from build123d import *

# Parameters (mm, degrees)
F0_W        = 73
F0_H        = 40
F1_DEPTH    = 26.5
F0_W_2      = 79
F0_H_2      = 42
F2_DEPTH    = 1.5
F3_W        = 12
F3_H        = 12
F4_DEPTH    = 2
F5_W        = 12
F5_H        = 12
F6_DEPTH    = 2
F7_T        = 2.5
F7_T3_DEPTH = 78
F7_T5_DEPTH = 45
F7_T7_DEPTH = 17
F7_T9_DEPTH = 17


# Not quite as in the source:
# - a shell that OpenCascade refuses in one call is made with other operations: the cavity is built on its own and cut out


with BuildPart() as f1:
    # F0 (on Front) → F1 (new body)
    with BuildSketch(Plane.XZ):
        Rectangle(F0_W, F0_H)
    extrude(amount=F1_DEPTH)

    # F0 (on Front) → F2 (join)
    with BuildSketch(Plane.XZ):
        Rectangle(F0_W_2, F0_H_2)
        Rectangle(F0_W, F0_H, mode=Mode.SUBTRACT)
    extrude(amount=F2_DEPTH)

    # F3 (on face) → F4 (join)
    with BuildSketch(Plane(origin=(-36.5, 0, 0), x_dir=(0, -1, 0), z_dir=(-1, 0, 0))):
        with Locations((7.75, 0)):
            Rectangle(F3_W, F3_H)
    extrude(amount=F4_DEPTH)

    # F5 (on face) → F6 (join)
    with BuildSketch(Plane.YZ.offset(36.5)):
        with Locations((-7.75, 0)):
            Rectangle(F5_W, F5_H)
    extrude(amount=F6_DEPTH)

    # F7: shell of thickness 2.5, made by hand


with BuildPart() as f7_core1:
    # F7_t2: copy of F1
    add(f1.part)

    # the walls: a layer under each face that stays
    f7_faces = [f7_core1.faces().sort_by_distance(p)[0] for p in [
        (0, -14, -20),
        (-36.8666666667, -1.5, -19.6),
        (36.5, -14, 0),
        (-36.5, -14, 0),
        (0, -0.75, -21),
        (39.5, -0.75, 0),
        (0, -0.75, 21),
        (-39.5, -0.75, 0),
        (0, -14, 20),
        (37.5, -13.75, 0),
        (37.5, -7.75, 6),
        (37.5, -1.75, 0),
        (37.5, -7.75, -6),
        (-37.5, -1.75, 0),
        (-37.5, -7.75, 6),
        (-37.5, -13.75, 0),
        (-37.5, -7.75, -6),
        (0, 0, 0),
        (38.5, -7.75, 0),
        (-38.5, -7.75, 0),
    ]]
    thicken(f7_faces, amount=-F7_T, mode=Mode.SUBTRACT)

    # F7_s4 → F7_t3 (cut)
    with BuildSketch(Plane.YZ.offset(-39)):
        Polygon((-1.525, -20.025), (-1.5, -17.5), (1, -17.5), (1, -20), align=None)
        Polygon((-1.525, 20.025), (1, 20), (1, 17.5), (-1.5, 17.5), align=None)
    extrude(amount=F7_T3_DEPTH, mode=Mode.SUBTRACT)

    # F7_s6 → F7_t5 (cut)
    with BuildSketch(Plane.XY.offset(-22.5)):
        Polygon((36.525, -1.525), (36.5, 1), (34, 1), (34, -1.5), align=None)
        Polygon((-36.525, -1.525), (-36.5, 1), (-34, 1), (-34, -1.5), align=None)
    extrude(amount=F7_T5_DEPTH, mode=Mode.SUBTRACT)

    # F7_s8 → F7_t7 (cut)
    with BuildSketch(Plane.XY.offset(-8.5)):
        Polygon((36.525, -13.775), (34, -13.75), (34, -11.25), (36.5, -11.25), align=None)
        Polygon((36.525, -1.725), (34, -1.75), (34, -4.25), (36.5, -4.25), align=None)
        Polygon((-36.525, -1.725), (-34, -1.75), (-34, -4.25), (-36.5, -4.25), align=None)
        Polygon((-36.525, -13.775), (-34, -13.75), (-34, -11.25), (-36.5, -11.25), align=None)
    extrude(amount=F7_T7_DEPTH, mode=Mode.SUBTRACT)

    # F7_s10 → F7_t9 (cut)
    with BuildSketch(Plane.XZ.offset(-0.75)):
        Polygon((36.525, 6.025), (34, 6), (34, 3.5), (36.5, 3.5), align=None)
        Polygon((36.525, -6.025), (34, -6), (34, -3.5), (36.5, -3.5), align=None)
        Polygon((-36.525, 6.025), (-34, 6), (-34, 3.5), (-36.5, 3.5), align=None)
        Polygon((-36.525, -6.025), (-34, -6), (-34, -3.5), (-36.5, -3.5), align=None)
    extrude(amount=F7_T9_DEPTH, mode=Mode.SUBTRACT)


with BuildPart() as f1_1:
    add(f1.part)

    # what is left inside the walls is the cavity
    f7_cavity = [f7_core1.part.solids().sort_by_distance(p)[0] for p in [
        (0, -2.525, -5.833333),
    ]]
    add(f7_cavity, mode=Mode.SUBTRACT)


solid = f1_1.part
Can you work these out from the model? Positions are in its coordinate system, mm. A direction names the side the tool comes from. Round coordinates to 2 decimals unless told otherwise and drop trailing zeros. Loops run counter-clockwise (first coordinate to the right, second up) from the corner with the lowest first, then second, coordinate; pieces in that order, holes last. Notation, with made-up numbers: (-12, -30.75) - (-3, -30.75) arc R25 cw to (-3, 2.25) - close; hole circle Ø4 at (3.5, 47). An arc over 180 degrees is marked (long way). Answer in a Markdown table with one row per item. Add a question column.
Q1. For pin 1 Ø8 at (x, y) = (12, -10.5) entering from +Z; pin 2 Ø1 at (y, z) = (-23, 15) entering from -X; pin 3 Ø2 at (x, z) = (37.5, -1.5) entering from +Y; pin 4 Ø0.6 at (x, y) = (-37, -10) entering from +Z, each with a flat end and sliding along its axis, tell me the tip position at first contact or that it passes through.
Q2. I want a section at A-A on x = -28. List the corners of the cut face in (y, z) for me, and give its area (3 significant figures).
Q3. I need wall thicknesses on L1, parallel to X at y = -12, z = 12; L2, parallel to Z at x = 3, y = -10.25; L3, parallel to X at y = -13, z = 5.5. Which ranges of each line are inside material? Lowest first, please.
Q4. We'd pull the mould along Y, two halves only. Please class faces 1 (the flat face through (0, -2.5, 0)), 2 (the flat face through (-35, -11.25, 0)), 3 (the flat face through (-1, -1, -21)): pulls with the +Y half, pulls with the -Y half, needs draft (parallel to the pull), parting line crosses it, or undercut.
Q5. I want a section at D-D on y = -3.25. List the corners of the cut face in (x, z) for me.
Q6. Which directions (+Z, -Z, +X, -X, +Y, -Y) give clear straight access to the entire face, cutting with the end or side of a thin tool? Please do faces 4 (the flat face through (38.5, -8, 0)), 5 (the flat face through (0, -14, -17.5)), 6 (the flat face through (-37, -8, -6)), 7 (the flat face through (-37, -13.75, 0)), 8 (the flat face through (-35, -8, 3.5)).
Q7. I want a section at C-C on z = 0. List the corners of the cut face in (x, y) for me.
Q8. I want a section at B-B on y = -15. List the corners of the cut face in (x, z) for me, and give its area (3 significant figures).
A:
| question | item | result |
|---|---|---|
| 1 | pin 1 | z = 20 |
| 1 | pin 2 | x = -36.5 |
| 1 | pin 3 | y = 0 |
| 1 | pin 4 | z = 6 |
| 2 | outline | (-26.5, -20) - (-1.5, -20) - (-1.5, -21) - (0, -21) - (0, 21) - (-1.5, 21) - (-1.5, 20) - (-26.5, 20) - (-26.5, 17.5) - (-2.5, 17.5) - (-2.5, -17.5) - (-26.5, -17.5) - close |
| 2 | area | 223 mm^2 |
| 3 | L1 | -36.5 to -34, 34 to 36.5 |
| 3 | L2 | -20 to -17.5, 17.5 to 20 |
| 3 | L3 | -38.5 to -34, 34 to 38.5 |
| 4 | face 1 | pulls with the -Y half |
| 4 | face 2 | undercut |
| 4 | face 3 | needs draft |
| 5 | outline | (-38.5, -6) - (-36.5, -6) - (-36.5, -20) - (36.5, -20) - (36.5, -6) - (38.5, -6) - (38.5, 6) - (36.5, 6) - (36.5, 20) - (-36.5, 20) - (-36.5, 6) - (-38.5, 6) - close; hole (-34, -17.5) - (34, -17.5) - (34, 17.5) - (-34, 17.5) - close |
| 6 | face 4 | +Z, -Z, +X, -Y |
| 6 | face 5 | -Y |
| 6 | face 6 | -Z, -X, -Y |
| 6 | face 7 | +Z, -Z, -X, -Y |
| 6 | face 8 | none |
| 7 | outline | (-39.5, -1.5) - (-36.5, -1.5) - (-36.5, -1.75) - (-38.5, -1.75) - (-38.5, -13.75) - (-36.5, -13.75) - (-36.5, -26.5) - (-34, -26.5) - (-34, -11.25) - (-36, -11.25) - (-36, -4.25) - (-34, -4.25) - (-34, -2.5) - (34, -2.5) - (34, -4.25) - (36, -4.25) - (36, -11.25) - (34, -11.25) - (34, -26.5) - (36.5, -26.5) - (36.5, -13.75) - (38.5, -13.75) - (38.5, -1.75) - (36.5, -1.75) - (36.5, -1.5) - (39.5, -1.5) - (39.5, 0) - (-39.5, 0) - close |
| 8 | outline | (-36.5, -20) - (36.5, -20) - (36.5, 20) - (-36.5, 20) - close; hole (-34, -17.5) - (34, -17.5) - (34, 17.5) - (-34, 17.5) - close |
| 8 | area | 540 mm^2 |
